For this review, take the finished solid that the model builds, in its own axes (mm). Round coordinates to 2 decimals unless told otherwise and drop trailing zeros. Loops run counter-clockwise (first coordinate to the right, second up) from the corner with the lowest first, then second, coordinate; pieces in that order, holes last.
```python
from build123d import *

# Parameters (mm, degrees)
BOSS_EXTRUDE2_DEPTH = 4


with BuildPart() as part:
    # 3DSketch1 → Boss-Extrude2 (new body)
    with BuildSketch(Plane(origin=(-135.319434073, -27.39955072, -28.163146814), x_dir=(-1.1839737659606398e-15, -0.03268810373539661, 0.9994656011460245), z_dir=(-1, 0, 0))):
        Polygon((0, 0), (3.028470594, 24.815889383), (-0.942071707, 25.300444678), (1.480704768, 45.153156184), (5.451247069, 44.668600889), (8.479717663, 69.484490272), (14.435531115, 68.757657329), (14.92008641, 72.728199631), (34.772797916, 70.305423155), (34.288242621, 66.334880854), (44.214598374, 65.123492617), (44.699153669, 69.094034918), (64.551865176, 66.671258443), (64.067309881, 62.700716141), (73.993665634, 61.489327904), (76.223321536, 51.741064748), (80.122626798, 52.632927109), (82.3522827, 42.884663953), (78.452977438, 41.992801592), (80.68263334, 32.244538436), (84.581938602, 33.136400797), (83.663812307, 29.243195934), (93.396824464, 26.947880195), (94.31495076, 30.841085058), (108.914468996, 27.398111451), (107.996342701, 23.504906588), (117.729354858, 21.209590849), (118.647481154, 25.102795712), (133.24699939, 21.659822105), (132.328873095, 17.766617242), (142.061885253, 15.471301504), (142.980011548, 19.364506367), (157.579529784, 15.921532759), (156.661403489, 12.028327896), (162.501210784, 10.651138453), (160.205895045, 0.918126295), (164.099099908, 0), (161.80378417, -9.733012158), (157.910579307, -8.814885862), (155.615263569, -18.54789802), align=None)
    extrude(amount=-BOSS_EXTRUDE2_DEPTH)


solid = part.part
```
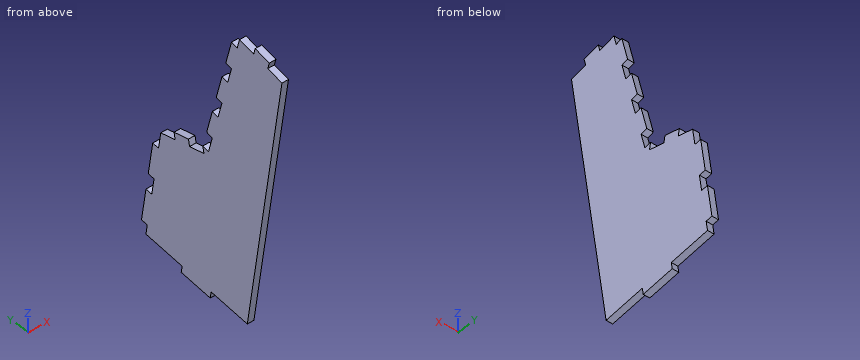
(1) Insertion check: pin 1 Ø1 at (x, z) = (-132, 58.5) entering from +Y. The pin has a flat end and moves straight along its axis. Give the tip position at first contact, or say it passes through.
(2) Add section A-A (z = 121). Give the boundary of the cut face in (x, y), plus the area to 3 significant figures.
(3) For L1, parallel to Y at x = -134.1, z = 45.5; L2, parallel to Y at x = -135, z = 0; L3, parallel to Z at x = -132.2, y = 30, list the stretches that pass through material, from the lowest coordinate up.
(4) Add section B-B (y = -37.5). Give the boundary of the cut face in (x, z), plus the area to 3 significant figures.
Outcome:
1. pin 1: stops at y = -1.34
2. outline: (-135.32, -50.15) - (-131.32, -50.15) - (-131.32, -14.24) - (-135.32, -14.24) - close
2. area: 144 mm2
3. L1: y = -38.63 to 32
3. L2: y = -31.69 to 43.11
3. L3: z = -19.25 to 48.12
4. outline: (-135.32, 38.07) - (-131.32, 38.07) - (-131.32, 134.57) - (-135.32, 134.57) - close
4. area: 386 mm2
